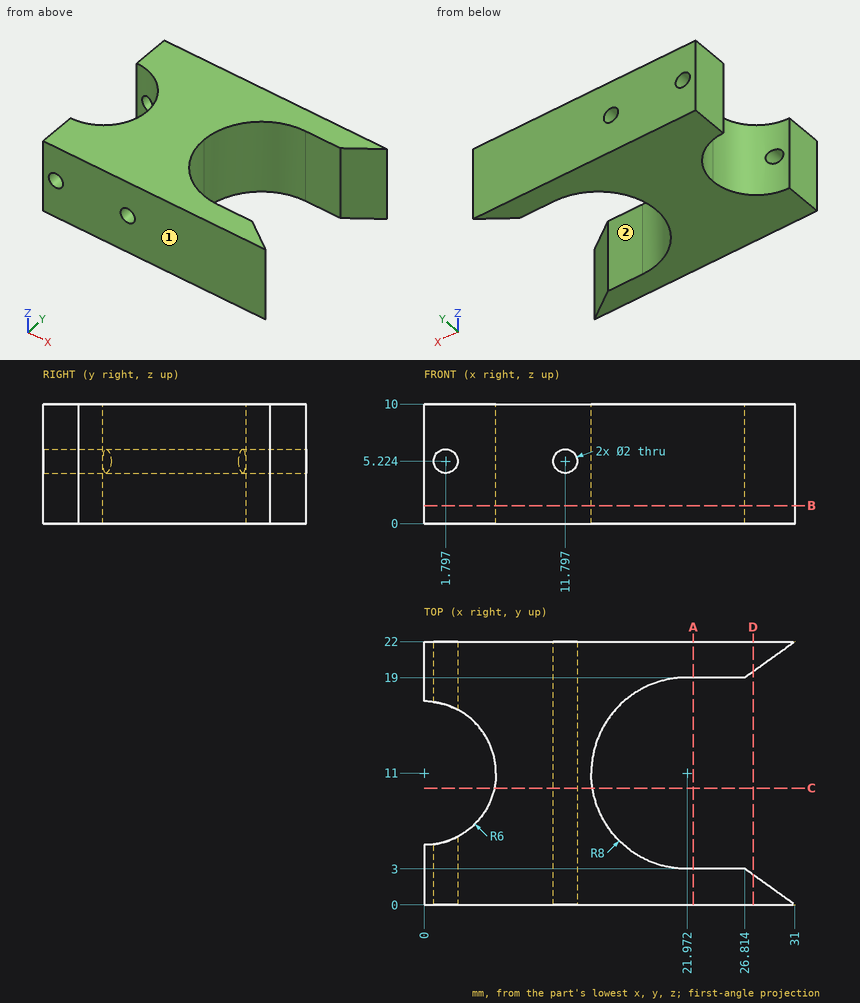
Design review of the part shown in the three views and the two pictorial views. Dimensions are in mm from the part's minimum x, y and z. A direction names the side the tool comes from. Coordinates: 2 decimals unless noted, no trailing zeros. Order: outer loops, then holes, each group sorted by start corner. A loop starts at its lowest first (then second) coordinate and runs counter-clockwise, first axis right, second up. Notation, with made-up numbers: (-35.5, 75) - (15.5, 75) arc R28 cw to (15.5, 107) - close; hole circle Ø6 at (56.25, 40.25). An arc over 180 degrees is marked (long way). Answer as CSV lines item,"result". Start each with the question number.
1) Add section C-C (y = 9.75). State the section outline as (x, z) points (1 decimal).
2) Add section B-B (z = 1.5). State the section outline as (x, y) points, then the cut area to 3 significant figures.
3) Add section D-D (x = 27.5). State the section outline as (y, z) points.
4) Machinability: for the marked faces 1 and 2, which of the approach directions +Z, -Z, +X, -X, +Y, -Y give a long, thin tool a straight path to every point of the face, cutting with its end or side? Answer none if there is none.
5) To check wall thickness, follow line 1 along Z through (x, y) = (12, 19.25) (1 decimal); line 2 along Z through (x, y) = (11, 16.75) (1 decimal); line 3 along X through (y, z) = (11.75, 5.75) (1 decimal). State the ranges of each line that lie inside material, in increasing order. Write a range as [from, to].
6) Insertion check: P1, Ø2.5, axis at x = 1.8, z = 5.22, coming from the -Y side. The pin has a flat end and moves straight along its axis. Give the tip position at first contact, or say it passes through.
7) Add section A-A (x = 22.5). State the section outline as (y, z) points, then the cut area to 3 significant figures.
Result:
1,outline,"(5.9, 0) - (14.1, 0) - (14.1, 10) - (5.9, 10) - close; hole circle Ø2 at (11.8, 5.2)"
2,outline,"(0, 0) - (31, 0) - (26.81, 3) - (21.97, 3) arc R8 cw to (21.97, 19) - (26.81, 19) - (31, 22) - (0, 22) - (0, 17) arc R6 cw to (0, 5) - close"
2,area,"368 mm^2"
3,outline,"(0, 0) - (2.51, 0) - (2.51, 10) - (0, 10) - close; (19.49, 0) - (22, 0) - (22, 10) - (19.49, 10) - close"
4,face 1,"+Z, -Z, +X, -X, -Y"
4,face 2,"+Z, -Z, +X"
5,line 1,"[0, 4.2], [6.2, 10]"
5,line 2,"[0, 4.6], [5.8, 10]"
5,line 3,"[6, 10.9], [12.6, 14]"
6,P1,"y = 0"
7,outline,"(0, 0) - (3, 0) - (3, 10) - (0, 10) - close; (19, 0) - (22, 0) - (22, 10) - (19, 10) - close"
7,area,"60.0 mm^2"
